```python
from build123d import *

# Parameters (mm, degrees)
ESQUISSE1_R             = 11
ESQUISSE1_R_2           = 4
BOSS_EXTRU_1_DEPTH      = 3.5
ESQUISSE2_R             = 9.3
ESQUISSE2_R_2           = 5.7
ENL_V_MAT_EXTRU_1_DEPTH = 0.2


with BuildPart() as part:
    # Esquisse1 → Boss.-Extru.1 (new, symmetric)
    with BuildSketch(Plane(origin=(0, 0, 0), x_dir=(0, 0, -1), z_dir=(1, 0, 0))):
        Circle(ESQUISSE1_R)
        Circle(ESQUISSE1_R_2, mode=Mode.SUBTRACT)
    extrude(amount=BOSS_EXTRU_1_DEPTH, both=True)

    # Esquisse2 → Enlèv. mat.-Extru.1 (cut)
    with BuildSketch(Plane(origin=(3.5, 0, 0), x_dir=(0, 0, -1), z_dir=(1, 0, 0))):
        Circle(ESQUISSE2_R)
        Circle(ESQUISSE2_R_2, mode=Mode.SUBTRACT)
    enl_v_mat_extru_1 = extrude(amount=-ENL_V_MAT_EXTRU_1_DEPTH, mode=Mode.SUBTRACT)

    # Symétrie1: Enlèv. mat.-Extru.1 across plane
    add(enl_v_mat_extru_1.mirror(Plane(origin=(0, 0, 0), x_dir=(0, 0, 1), z_dir=(1, 0, 0))), mode=Mode.SUBTRACT)


solid = part.part
```
Design review of the part built by this model. Coordinates are the model's own, in mm. A direction names the side the tool comes from. Coordinates: 2 decimals unless noted, no trailing zeros. Order: outer loops, then holes, each group sorted by start corner. A loop starts at its lowest first (then second) coordinate and runs counter-clockwise, first axis right, second up. Notation, with made-up numbers: (3, 55.5) -> (46, 55.5) arc R14 ccw to (46, 59.5) -> close; hole circle Ø7 at (-20.5, 55.5). An arc over 180 degrees is marked (long way). One line per item, written item: value. Start each with the question number.
Q1. For probe 1 along Y at (x, z) = (3.45, 0); probe 2 along Y at (x, z) = (0.75, 0); probe 3 along Z at (x, y) = (1.5, 1), list the stretches that pass through material, from the lowest coordinate up.
Q2. Insertion check: pin 1 Ø3 at (x, z) = (0, -7) entering from +Y; pin 2 Ø1.5 at (x, z) = (-0.5, 2) entering from -Y; pin 3 Ø4 at (x, y) = (-1, 8) entering from -Z. Each pin has a flat end and moves straight along its axis. Give the tip position at first contact, or say it passes through.
Q3. Mouldability with a two-part tool opening along Z and no side actions: class faces 1 (the cylindrical face through (-0.049, -3.905, 0.867)), 2 (the cylindrical face through (0.05, -10.74, 2.38)), 3 (the flat face through (3.5, 4.9, 8.2)) as pulls with the +Z half, pulls with the -Z half, needs draft (parallel to the pull), parting line crosses it, or undercut.
Q4. Tool access review of faces 4 (the flat face through (-3.3, 4.3, -4)), 5 (the flat face through (-3.5, -4, -2)), 6 (the flat face through (3.3, 4.3, -4)): name each direction out of +Z, -Z, +X, -X, +Y, -Y from which nothing blocks a thin tool from reaching the whole face with its end or side.
Q5. Take a section at A-A, the plane z = 0. State the section outline as (x, y) points.
Q6. Take a section at C-C, the plane x = 0.5. State the section outline as (y, z) points, then the cut area to 3 significant figures.
Q7. Take a section at D-D, the plane y = 4.75. State the section outline as (x, z) points.
Values follow:
1. probe 1: y = -11 to -9.3, -5.7 to -4, 4 to 5.7, 9.3 to 11
1. probe 2: y = -11 to -4, 4 to 11
1. probe 3: z = -10.95 to -3.87, 3.87 to 10.95
2. pin 1: stops at y = 9.53
2. pin 2: stops at y = -10.93
2. pin 3: stops at z = -9.22
3. face 1: undercut
3. face 2: parting line crosses it
3. face 3: needs draft
4. face 4: -X
4. face 5: +Z, -Z, -X, +Y, -Y
4. face 6: +X
5. outline: (-3.5, -11) -> (3.5, -11) -> (3.5, -9.3) -> (3.3, -9.3) -> (3.3, -5.7) -> (3.5, -5.7) -> (3.5, -4) -> (-3.5, -4) -> (-3.5, -5.7) -> (-3.3, -5.7) -> (-3.3, -9.3) -> (-3.5, -9.3) -> close; (-3.5, 4) -> (3.5, 4) -> (3.5, 5.7) -> (3.3, 5.7) -> (3.3, 9.3) -> (3.5, 9.3) -> (3.5, 11) -> (-3.5, 11) -> (-3.5, 9.3) -> (-3.3, 9.3) -> (-3.3, 5.7) -> (-3.5, 5.7) -> close
6. outline: circle Ø22 at (0, 0); hole circle Ø8 at (0, 0)
6. area: 330 mm2
7. outline: (-3.5, -9.92) -> (3.5, -9.92) -> (3.5, -8) -> (3.3, -8) -> (3.3, -3.15) -> (3.5, -3.15) -> (3.5, 3.15) -> (3.3, 3.15) -> (3.3, 8) -> (3.5, 8) -> (3.5, 9.92) -> (-3.5, 9.92) -> (-3.5, 8) -> (-3.3, 8) -> (-3.3, 3.15) -> (-3.5, 3.15) -> (-3.5, -3.15) -> (-3.3, -3.15) -> (-3.3, -8) -> (-3.5, -8) -> close
